Autodesk Fusion 360 part; units mm, degrees
sketch "Sketch1" plane through (0, 0, 0) normal (0, 1, 0) x (1, 0, 0)
  line L0 (0, 0) -> (20.5, 0)
  line L1 (20.5, 0) -> (20.5, -20.5)
  line L2 (20.5, -20.5) -> (0, -20.5)
  line L3 (0, -20.5) -> (0, 0)
  line L4 (0, 0) -> (-4, 0)
  line L5 (-4, 0) -> (-4, 4)
  line L6 (-4, 4) -> (0, 4)
  line L7 (0, 4) -> (0, 0)
  line L8 (-4, 4) -> (24.5, 4)
  line L9 (24.5, 4) -> (24.5, -24.5)
  line L10 (24.5, -24.5) -> (-4, -24.5)
  line L11 (-4, -24.5) -> (-4, 4)
  dimension "d1" = 20.5
  dimension "d2" = 20.5
  dimension "d3" = 4
  dimension "d4" = 4
  dimension "d5" = 28.5
  dimension "d6" = 28.5
extrude "Extrude1" add sketch "Sketch1" along normal blind 20
chamfer "Chamfer1" distance 3 angle 45 5 edges at (24.5, 20, 10.25) (10.25, 20, 24.5) (24.5, 10, 24.5) (24.5, 0, 10.25) (10.25, 0, 24.5)
sketch "Sketch2" plane through (0, 0, -4) normal (0, 0, -1) x (-1, 0, 0)
  line L0 (-24.5, 3) -> (-21.5, 0)
  line L1 (-21.5, 0) -> (4, 0)
  line L2 (4, 0) -> (4, 20)
  line L3 (4, 20) -> (-21.5, 20)
  line L4 (-21.5, 20) -> (-24.5, 17)
  line L5 (-24.5, 17) -> (-24.5, 3)
  line L6 (-24.5, 10) -> (-10.25, 10)
  line L7 (-7.6519, 5.5) -> (-5.0538, 10)
  line L8 (-5.0538, 10) -> (-7.6519, 14.5)
  line L9 (-7.6519, 14.5) -> (-12.8481, 14.5)
  line L10 (-12.8481, 14.5) -> (-15.4462, 10)
  line L11 (-15.4462, 10) -> (-12.8481, 5.5)
  line L12 (-12.8481, 5.5) -> (-7.6519, 5.5)
  point P0 (-10.25, 10)
  dimension "d10" = 14.25
  dimension "d11" = 4.5
extrude "Extrude2" add sketch "Sketch2" along normal blind 4
sketch "Sketch3" plane through (0, 0, -8) normal (0, 0, -1) x (-1, 0, 0)
  line L0 (-7.6519, 5.5) -> (-12.8481, 5.5)
  line L1 (-15.4462, 10) -> (-12.8481, 14.5)
  line L2 (-12.8481, 14.5) -> (-7.6519, 14.5)
  line L3 (-7.6519, 14.5) -> (-5.0538, 10)
  line L4 (-5.0538, 10) -> (-7.6519, 5.5)
  line L5 (-24.5, 17) -> (-24.5, 3)
  line L6 (-24.5, 3) -> (-21.5, 0)
  line L7 (-21.5, 0) -> (4, 0)
  line L8 (4, 0) -> (4, 20)
  line L9 (4, 20) -> (-21.5, 20)
  line L10 (-21.5, 20) -> (-24.5, 17)
  line L11 (-7.6519, 14.5) -> (-5.0538, 14.5)
  line L12 (-5.0538, 14.5) -> (-5.0538, 10)
  line L13 (-15.4462, 10) -> (-15.4462, 14.5)
  line L14 (-15.4462, 14.5) -> (-12.8481, 14.5)
extrude "Extrude3" cut sketch "Sketch3" against normal blind 4 contours L1 L13 L14 | L3 L11 L12
sketch "Sketch4" plane through (0, 0, -8) normal (0, 0, -1) x (-1, 0, 0)
  line L0 (-15.4462, 14.5) -> (-5.0538, 14.5)
  line L1 (-5.0538, 14.5) -> (-5.0538, 10)
  line L2 (-5.0538, 10) -> (-7.6519, 5.5)
  line L3 (-7.6519, 5.5) -> (-12.8481, 5.5)
  line L4 (-12.8481, 5.5) -> (-15.4462, 10)
  line L5 (-15.4462, 10) -> (-15.4462, 14.5)
  line L6 (-24.5, 17) -> (-24.5, 3)
  line L7 (-24.5, 3) -> (-21.5, 0)
  line L8 (-21.5, 0) -> (4, 0)
  line L9 (4, 0) -> (4, 20)
  line L10 (4, 20) -> (-21.5, 20)
  line L11 (-21.5, 20) -> (-24.5, 17)
  line L12 (-10.25, 5.5) -> (-10.25, 10)
  circle A0 centre (-10.25, 10) radius 2
  line L13 (-5.0538, 14.5) -> (-15.4186, 14.5)
  line L14 (-15.4186, 14.5) -> (-15.4186, 5.5)
  line L15 (-15.4186, 5.5) -> (-5.0538, 5.5)
  line L16 (-5.0538, 5.5) -> (-5.0538, 14.5)
  line L17 (7, 22) -> (-27, 22)
  line L18 (-27, 22) -> (-27, -2)
  line L19 (-27, -2) -> (7, -2)
  line L20 (7, -2) -> (7, 22)
  dimension "d16" = 4
extrude "Extrude4" add sketch "Sketch4" along normal blind 5 contours L0 L1 L2 L3 L4 L13 L14 L15 L16 | L4 L14 L15 | L2 L15 L16 | L6 L7 L8 L9 L10 L11
extrude "Extrude5" add 1 faces at (0.0833, 10, -13) along direction (0, 0, -1) blind 1.75
sketch "Sketch5" plane through (-4, 0, 0) normal (-1, 0, 0) x (0, 0, 1)
  line L0 (21.5, 0) -> (24.5, 3)
  line L1 (24.5, 3) -> (24.5, 17)
  line L2 (24.5, 17) -> (21.5, 20)
  line L3 (21.5, 20) -> (-14.75, 20)
  line L4 (-14.75, 20) -> (-14.75, 0)
  line L5 (-14.75, 0) -> (21.5, 0)
  line L6 (-14.75, 20) -> (-4.75, 20)
  line L7 (-4.75, 20) -> (-4.75, 0)
  line L8 (-4.75, 0) -> (-14.75, 0)
  line L9 (-14.75, 0) -> (-14.75, 20)
  dimension "d21" = 10
extrude "Extrude6" add sketch "Sketch5" along normal blind 15 contours L3 L4 L5 L6 L7 L8 L9
sketch "Sketch6" plane through (0, 0, -4.75) normal (0, 0, 1) x (1, 0, 0)
  line L0 (-4, 0) -> (-4, 20)
  line L1 (-4, 20) -> (-19, 20)
  line L2 (-19, 20) -> (-19, 0)
  line L3 (-19, 0) -> (-4, 0)
  line L4 (-19, 10) -> (-11.5, 10)
  circle A0 centre (-11.5, 10) radius 3.5
  dimension "d24" = 7.5
  dimension "d25" = 7
extrude "Extrude7" cut sketch "Sketch6" against normal blind 10 contours A0
sketch "Sketch7" plane through (0, 0, 0) normal (0, -1, 0) x (1, 0, 0)
  line L0 (21.5, -14.75) -> (21.5, 21.5)
  line L1 (21.5, 21.5) -> (-4, 21.5)
  line L2 (-4, 21.5) -> (-4, -4.75)
  line L3 (-4, -4.75) -> (-19, -4.75)
  line L4 (-19, -4.75) -> (-19, -14.75)
  line L5 (-19, -14.75) -> (21.5, -14.75)
  line L6 (0, 20.5) -> (20.5, 20.5)
  line L7 (20.5, 20.5) -> (20.5, 0)
  line L8 (20.5, 0) -> (0, 0)
  line L9 (0, 0) -> (0, 20.5)
  line L10 (-19, -4.75) -> (-19, 10.25)
  circle A0 centre (-19, 10.25) radius 15
  dimension "d28" = 15
extrude "Extrude8" add sketch "Sketch7" against normal blind 20 contours L2 L3 A0
sketch "Sketch8" plane through (0, 0, -14.75) normal (0, 0, -1) x (-1, 0, 0)
  circle A0 centre (11.5, 10) radius 3.5
  line L0 (-15.4462, 14.5) -> (-15.4186, 14.5)
  line L1 (-15.4186, 14.5) -> (-15.4186, 9.9523)
  line L2 (-15.4186, 9.9523) -> (-15.4462, 10)
  line L3 (-15.4462, 10) -> (-15.4462, 14.5)
  circle A1 centre (-10.25, 10) radius 2
  line L4 (-21.5, 20) -> (-24.5, 17)
  line L5 (-24.5, 17) -> (-24.5, 3)
  line L6 (-24.5, 3) -> (-21.5, 0)
  line L7 (-21.5, 0) -> (19, 0)
  line L8 (19, 0) -> (19, 20)
  line L9 (19, 20) -> (-21.5, 20)
  circle A2 centre (11.5, 10) radius 5
  dimension "d31" = 10
extrude "Extrude9" cut sketch "Sketch8" along normal blind -10 and the other way blind 27 contours A2
extrude "Extrude10" cut 1 faces at (-11.9678, 9.7747, -4.75) along direction (0, 0, 1) blind 20
sketch "Sketch9" plane through (0, 0, -4.75) normal (0, 0, 1) x (1, 0, 0)
  circle A0 centre (-11.5, 10) radius 3.5
  circle A1 centre (-11.5, 10) radius 5
  circle A2 centre (-11.5, 10) radius 2
  dimension "d38" = 4
extrude "Extrude11" add sketch "Sketch9" against normal blind 10 contours A0
sketch "Sketch10" plane through (0, 0, -4) normal (0, 0, -1) x (-1, 0, 0)
  line L0 (-7.6519, 5.5) -> (-5.0538, 10)
  line L1 (-5.0538, 10) -> (-5.0538, 14.5)
  line L2 (-5.0538, 14.5) -> (-15.4462, 14.5)
  line L3 (-15.4462, 14.5) -> (-15.4462, 10)
  line L4 (-15.4462, 10) -> (-12.8481, 5.5)
  line L5 (-12.8481, 5.5) -> (-7.6519, 5.5)
  line L6 (-10.25, 5.5) -> (-10.25, 10)
  circle A0 centre (-10.25, 10) radius 2
  dimension "d41" = 4
extrude "Extrude12" cut sketch "Sketch10" against normal blind 3.5 contours A0
extrude "Extrude13" add 1 faces at (9.7539, 10.3541, -0.5) along direction (0, 0, -1) blind 0.5
extrude "Extrude14" add 1 faces at (3.9949, 17.2826, -14.75) along direction (0, 0, -1) blind 1
sketch "Sketch11" plane through (0, 0, -4) normal (0, 0, -1) x (-1, 0, 0)
  circle A0 centre (-10.25, 10) radius 2
  line L0 (-7.6519, 5.5) -> (-5.0538, 10)
  line L1 (-5.0538, 10) -> (-5.0538, 14.5)
  line L2 (-5.0538, 14.5) -> (-15.4462, 14.5)
  line L3 (-15.4462, 14.5) -> (-15.4462, 10)
  line L4 (-15.4462, 10) -> (-12.8481, 5.5)
  line L5 (-12.8481, 5.5) -> (-7.6519, 5.5)
  line L6 (-8.5179, 7) -> (-6.7859, 10)
  line L7 (-6.7859, 10) -> (-8.5179, 13)
  line L8 (-8.5179, 13) -> (-11.9821, 13)
  line L9 (-11.9821, 13) -> (-13.7141, 10)
  line L10 (-13.7141, 10) -> (-11.9821, 7)
  line L11 (-11.9821, 7) -> (-8.5179, 7)
  line L12 (-6.7859, 10) -> (-13.7141, 10)
  line L13 (-13.7141, 10) -> (-13.7141, 13)
  line L14 (-13.7141, 13) -> (-6.7859, 13)
  line L15 (-6.7859, 13) -> (-6.7859, 10)
  point P0 (-10.25, 10)
  dimension "d48" = 3
  dimension "d49" = 3
extrude "Extrude15" add sketch "Sketch11" along normal blind 5
extrude "Extrude16" add 1 faces at (13.16, 11.2893, -4) along direction (0, 0, -1) blind 1.5
extrude "Extrude17" add 1 faces at (15.4278, 11.4841, -9) along direction (0, 0, -1) blind 6.75
Design review of the part built by this model. Coordinates are the model's own, in mm. A direction names the side the tool comes from. Coordinates: 2 decimals unless noted, no trailing zeros. Order: outer loops, then holes, each group sorted by start corner. A loop starts at its lowest first (then second) coordinate and runs counter-clockwise, first axis right, second up. Notation, with made-up numbers: (49.25, -29.75) - (53.25, -29.75) arc R15 ccw to (53.25, -14.75) - close; hole circle Ø2 at (66.5, 2.25). An arc over 180 degrees is marked (long way). Put each result on its own line as item: value.
1) Tool access review of faces 5 (the face through (0, 10, 10)), 6 (the face through (-6.505, 9.78, -2.093)), 7 (the face through (10, 13, -7)), 8 (the face through (10, 10, -1)): name each direction out of +Z, -Z, +X, -X, +Y, -Y from which nothing blocks a thin tool from reaching the whole face with its end or side.
Response values:
face 5: +Y, -Y
face 6: +Z
face 7: none
face 8: -Z
2) Take a section at D-D, the plane z = -12. Give the boundary of the cut face in (x, y), and give its area (3 significant figures).
Response values:
outline: (-19, 0) - (21.5, 0) - (24.5, 3) - (24.5, 17) - (21.5, 20) - (-19, 20) - close; hole circle Ø4 at (-11.5, 10); hole circle Ø4 at (10.25, 10)
area: 836 mm²
3) Wall thickness on L1, parallel to Y at x = 10.25, z = -14; L2, parallel to X at y = 10, z = -1.5; L3, parallel to Z at x = 2, y = 4: over which ranges is each line inside the solid? List them lowest first. Write a range as from..to.
Response values:
L1: y = 0..8, 12..20
L2: x = -6.5..8.25, 12.25..24.5
L3: z = -15.75..0, 20.5..24.5
4) Take a section at A-A, the plane x = 10.25. Give the boundary of the cut face in (y, z), and give its area (3 significant figures).
Response values:
outline: (0, -15.75) - (8, -15.75) - (8, -8) - (7, -8) - (7, -5.5) - (8, -5.5) - (8, -1) - (12, -1) - (12, -5.5) - (13, -5.5) - (13, -8) - (12, -8) - (12, -15.75) - (20, -15.75) - (20, 0) - (0, 0) - close; (0, 20.5) - (20, 20.5) - (20, 21.5) - (17, 24.5) - (3, 24.5) - (0, 21.5) - close
area: 322 mm²
5) The part is to be moulded in two halves that separate along Y. For faces 1 (the face through (1, 0, -5)), 2 (the face through (10, 7, -7)), 3 (the face through (6.786, 12, -7)), 4 (the face through (24.5, 10, 3)), say which applies: released by +Y, released by -Y, zero draft, split by the parting line, or undercut.
Response values:
face 1: released by -Y
face 2: undercut
face 3: undercut
face 4: zero draft
6) Take a section at C-C, the plane z = 17. Give the boundary of the cut face in (x, y).
Response values:
outline: (-4, 0) - (0, 0) - (0, 20) - (-4, 20) - close; (20.5, 0) - (21.5, 0) - (24.5, 3) - (24.5, 17) - (21.5, 20) - (20.5, 20) - close
7) Insertion check: P1, Ø10, axis at y = 7.5, z = 6.5, coming from the -X side; P2, Ø3.5, axis at x = -11.5, y = 10, coming from the -Z side; P3, Ø5, axis at y = 10.5, z = 13.5, coming from the -X side; P4, Ø5, axis at x = -10.5, y = 9.5, coming from the +Z side. Each pin has a flat end and moves straight along its axis. Give the tip position at first contact, or say it passes through.
Response values:
P1: stops at x = -6.82
P2: passes through
P3: stops at x = -4
P4: stops at z = -4.75
8) Take a section at B-B, the plane y = 8.75. Count the separate pieces of the cut face and the enclosed holes in it, and give its area (3 significant figures).
Response values:
separate pieces: 2
enclosed holes: 1
area: 826 mm²
